Input: dimensioned drawing with shaded views. Units: mm. Origin: part minimum x, y, z. A direction names the side the tool comes from. Give positions to 0.01 mm unless a question says otherwise; leave off trailing zeros. Loops run counter-clockwise (first coordinate to the right, second up) from the corner with the lowest first, then second, coordinate; pieces in that order, holes last.
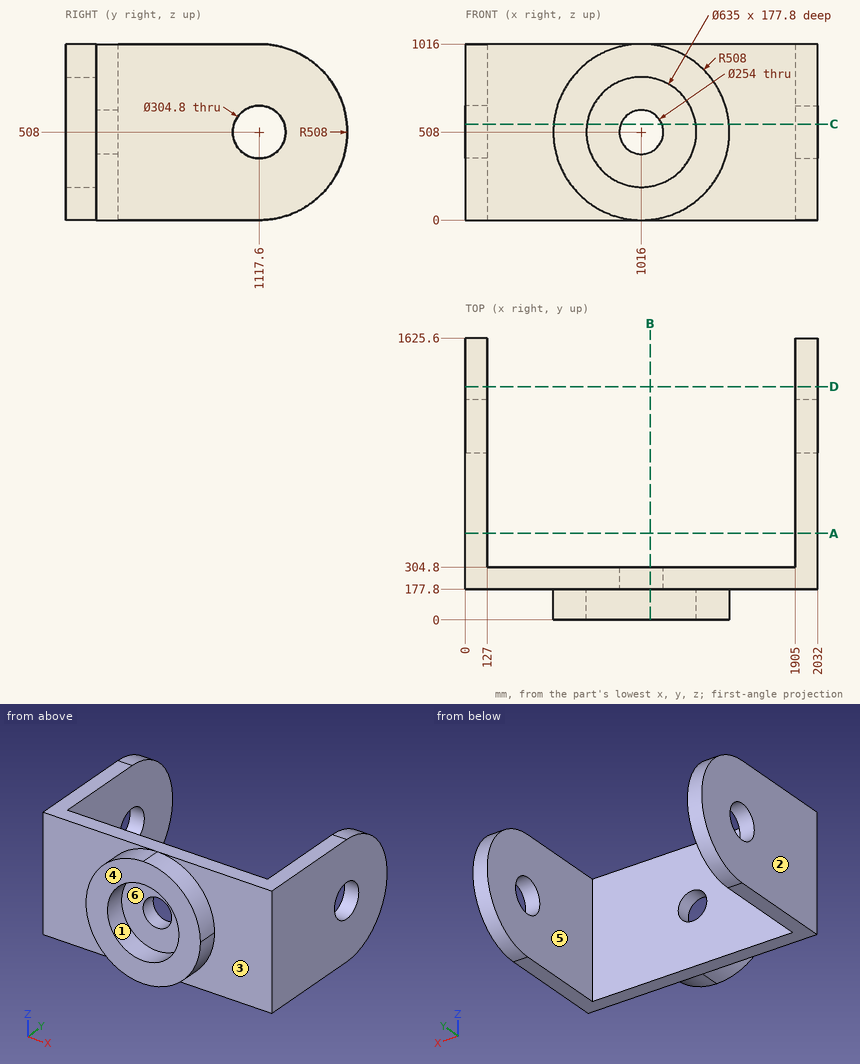
(1) First-contact query: pin 1 (3 mm diameter, centred on y = 264, z = 270, fed in from -X); pin 2 (10 mm diameter, centred on x = 902.5, z = 700, fed in from -Y); pin 3 (1 mm diameter, centred on x = 616, z = 866, fed in from +Y). Flat tips, straight axial feed; report the tip coordinate or a pass-through.
A:
pin 1: stops at x = 0
pin 2: stops at y = 177.8
pin 3: stops at y = 304.8
(2) Section D-D, the plane y = 1346. Return the cut outline in (x, z).
A:
outline: (0, 54.24) - (127, 54.24) - (127, 961.76) - (0, 961.76) - close; (1905, 54.24) - (2032, 54.24) - (2032, 961.76) - (1905, 961.76) - close
(3) Section C-C, the plane z = 553.5. Return the cut outline in (x, y).
A:
outline: (0, 177.8) - (510.04, 177.8) - (510.04, 0) - (701.78, 0) - (701.78, 177.8) - (897.43, 177.8) - (897.43, 304.8) - (127, 304.8) - (127, 972.15) - (0, 972.15) - close; (0, 1263.05) - (127, 1263.05) - (127, 1623.56) - (0, 1623.56) - close; (1134.57, 177.8) - (1330.22, 177.8) - (1330.22, 0) - (1521.96, 0) - (1521.96, 177.8) - (2032, 177.8) - (2032, 972.15) - (1905, 972.15) - (1905, 304.8) - (1134.57, 304.8) - close; (1905, 1263.05) - (2032, 1263.05) - (2032, 1623.56) - (1905, 1623.56) - close
(4) Reachability of the marked faces 4, 5 and 6 from +Z, -Z, +X, -X, +Y, -Y: full face, straight path, thin tool, end or side. Return the list, or none.
A:
face 4: +Z, -Z, +X, -X, -Y
face 5: +Z, -Z, +Y
face 6: -Y
(5) Section B-B, the plane x = 1067. Return the cut outline in (y, z).
A:
outline: (0, 2.57) - (177.8, 2.57) - (177.8, 0) - (304.8, 0) - (304.8, 391.69) - (177.8, 391.69) - (177.8, 194.62) - (0, 194.62) - close; (0, 821.38) - (177.8, 821.38) - (177.8, 624.31) - (304.8, 624.31) - (304.8, 1016) - (177.8, 1016) - (177.8, 1013.43) - (0, 1013.43) - close
(6) Ray query, line 1 along X through (y, z) = (406.5, 493); line 2 along Z through (x, y) = (1934, 1117.6); line 3 along Y through (x, z) = (597, 94.5). Return the intervals inside material, ascending.
A:
line 1: x = 0 to 127, 1905 to 2032
line 2: z = 0 to 355.6, 660.4 to 1016
line 3: y = 177.8 to 304.8
(7) Mould query, pull axis X, two halves, no side actions, for the marked faces 1, 2 and 3. Classes: pulls with the +X half, pulls with the -X half, needs draft (parallel to the pull), parting line crosses it, or undercut.
A:
face 1: undercut
face 2: pulls with the -X half
face 3: needs draft
(8) Section A-A, the plane y = 498.5. Return the cut outline in (x, z), then the cut area to 3 significant figures.
A:
outline: (0, 0) - (127, 0) - (127, 1016) - (0, 1016) - close; (1905, 0) - (2032, 0) - (2032, 1016) - (1905, 1016) - close
area: 258,000 mm2
